The model under review builds one solid part; all positions refer to its coordinate system, in mm. Face numbers are marked on the shaded views. A direction names the side the tool comes from. Give positions to 0.01 mm unless a question says otherwise; leave off trailing zeros. Order: outer loops, then holes, each group sorted by start corner. A loop starts at its lowest first (then second) coordinate and runs counter-clockwise, first axis right, second up. Notation, with made-up numbers: (22.5, -4) - (79.5, -4) arc R17 ccw to (79.5, 2) - close; hole circle Ø5 at (41, 2.5). An arc over 180 degrees is marked (long way). Use CSV: the item, a comma, the result in double quotes. Start each with the question number.
1. To check wall thickness, follow line 1 (X direction, y = 9.5, z = -12); line 2 (Y direction, x = -3.5, z = 8.5); line 3 (X direction, y = 6, z = 9.5). State the ranges of each line that lie inside material, in increasing order. Write a range as [from, to].
2. For pin 1 (0.9 mm diameter, centred on x = -0.5, z = 10, fed in from -Y); pin 2 (2 mm diameter, centred on x = 1.5, y = 7, fed in from -Z); pin 3 (1.5 mm diameter, centred on y = 7.5, z = -0.5, fed in from +X), all flat-tipped, find the tip position at first contact; note any pin that passes through.
3. Machinability: for the marked faces 1, 2 and 3, which of the approach directions +Z, -Z, +X, -X, +Y, -Y give a long, thin tool a straight path to every point of the face, cutting with its end or side? Answer none if there is none.
4. Take a section at D-D, the plane x = 2. State the section outline as (y, z) points.
5. Take a section at A-A, the plane z = 0. State the section outline as (x, y) points, then the cut area to 3 significant figures.
6. Take a section at B-B, the plane y = 8.5. State the section outline as (x, z) points.
7. Take a section at C-C, the plane x = 0. State the section outline as (y, z) points.
```python
from build123d import *

# Parameters (mm, degrees)
SKETCH_1_W          = 3
SKETCH_1_H          = 28
EXTRUDE_1_DEPTH     = 10
SKETCH_2_W          = 11
SKETCH_2_H          = 24
EXTRUDE_2_DEPTH     = 1.5
FILLET_1_R          = 1
SKETCH_3_W          = 11
SKETCH_3_H          = 36
EXTRUDE_3_DEPTH     = 1.5
FILLET_3_R          = 1
SKETCH_5_W          = 11
SKETCH_5_H          = 30
CUT_EXTRUDE_1_DEPTH = 6.5
CUT_EXTRUDE_2_DEPTH = 3
FILLET_4_R          = 2
FILLET_5_R          = 0.1


with BuildPart() as part:
    # Эскиз1 → Бобышка-Вытянуть1 (new body)
    with BuildSketch(Plane(origin=(0, 0, 0), x_dir=(1, 0, 0), z_dir=(0, 1, 0))):
        Rectangle(SKETCH_1_W, SKETCH_1_H)
    extrude(amount=EXTRUDE_1_DEPTH)

    # Эскиз2 → Бобышка-Вытянуть2 (add)
    with BuildSketch(Plane.XZ):
        Rectangle(SKETCH_2_W, SKETCH_2_H)
    extrude(amount=EXTRUDE_2_DEPTH)

    # Скругление1
    fillet_1_edges = [part.edges().sort_by_distance(p)[0] for p in [
        (-1.5, 5, -14),
        (1.5, 5, -14),
        (1.5, 5, 14),
        (-1.5, 5, 14),
    ]]
    fillet(fillet_1_edges, radius=FILLET_1_R)

    # Эскиз3 → Бобышка-Вытянуть3 (add)
    with BuildSketch(Plane(origin=(0, 10, 0), x_dir=(1, 0, 0), z_dir=(0, 1, 0))):
        Rectangle(SKETCH_3_W, SKETCH_3_H)
    extrude(amount=EXTRUDE_3_DEPTH)

    # Скругление3
    fillet_3_edges = [part.edges().sort_by_distance(p)[0] for p in [
        (5.5, -0.75, -12),
        (5.5, -0.75, 12),
        (-5.5, -0.75, 12),
        (-5.5, -0.75, -12),
    ]]
    fillet(fillet_3_edges, radius=FILLET_3_R)

    # Эскиз5 → Вырез-Вытянуть1 (cut)
    with BuildSketch(Plane(origin=(0, -1.5, 0), x_dir=(-1, 0, 0), z_dir=(0, -1, 0))):
        Rectangle(SKETCH_5_W, SKETCH_5_H)
    extrude(amount=-CUT_EXTRUDE_1_DEPTH, mode=Mode.SUBTRACT)

    # Эскиз6 → Вырез-Вытянуть2 (cut)
    with BuildSketch(Plane.XZ.offset(-5)):
        Polygon((-1.6, -10), (-0.360392927, -8.760392927), (-0.360392927, -8.250794149), (0.360392927, -8.250794149), (0.360392927, -8.760392927), (1.6, -10), (0.360392927, -11.239607073), (0.360392927, -11.788123746), (-0.360392927, -11.788123746), (-0.360392927, -11.239607073), align=None)
        Polygon((-0.360392927, 11.788123746), (0.360392927, 11.788123746), (0.360392927, 11.239607073), (1.6, 10), (0.360392927, 8.760392927), (0.360392927, 8.250794149), (-0.360392927, 8.250794149), (-0.360392927, 8.760392927), (-1.6, 10), (-0.360392927, 11.239607073), align=None)
    extrude(amount=-CUT_EXTRUDE_2_DEPTH, mode=Mode.SUBTRACT)

    # Скругление4
    fillet_4_edges = [part.edges().sort_by_distance(p)[0] for p in [
        (-5.5, 10.75, -18),
        (-5.5, 10.75, 18),
        (5.5, 10.75, 18),
        (5.5, 10.75, -18),
    ]]
    fillet(fillet_4_edges, radius=FILLET_4_R)

    # Скругление5
    fillet_5_edges = [part.edges().sort_by_distance(p)[0] for p in [
        (1.5, 6.5, 10.1),
        (1.5, 6.5, 9.9),
        (-1.5, 6.5, 9.9),
        (-1.5, 6.5, 10.1),
        (1.5, 6.5, -9.9),
        (1.5, 6.5, -10.1),
        (-1.5, 6.5, -10.1),
        (-1.5, 6.5, -9.9),
    ]]
    fillet(fillet_5_edges, radius=FILLET_5_R)


solid = part.part
```
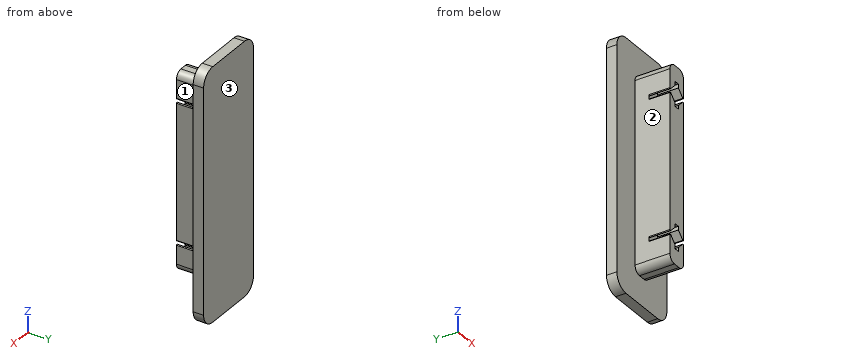
Determined:
1,line 1,"x = [-1.5, 1.5]"
1,line 2,"y = [10, 11.5]"
1,line 3,"x = [-1.5, -1.1], [1.1, 1.5]"
2,pin 1,"stops at y = 8"
2,pin 2,"stops at z = -14"
2,pin 3,"stops at x = 1.5"
3,face 1,"+Z, -Z, +X, -Y"
3,face 2,"+Z, -Z, -X, -Y"
3,face 3,"+Z, -Z, +X, -X, +Y"
4,outline,"(10, -18) - (11.5, -18) - (11.5, 18) - (10, 18) - close"
5,outline,"(-5.5, 10) - (-1.5, 10) - (-1.5, 5) - (1.5, 5) - (1.5, 10) - (5.5, 10) - (5.5, 11.5) - (-5.5, 11.5) - close"
5,area,"31.5 mm²"
6,outline,"(-1.5, -13) arc R1 ccw to (-0.5, -14) - (0.5, -14) arc R1 ccw to (1.5, -13) - (1.5, 13) arc R1 ccw to (0.5, 14) - (-0.5, 14) arc R1 ccw to (-1.5, 13) - close"
7,outline,"(5, -14) - (10, -14) - (10, -18) - (11.5, -18) - (11.5, 18) - (10, 18) - (10, 14) - (5, 14) - (5, 11.79) - (8, 11.79) - (8, 8.25) - (5, 8.25) - (5, -8.25) - (8, -8.25) - (8, -11.79) - (5, -11.79) - close"
